For this review, take the finished solid that the model builds, in its own axes (mm). A direction names the side the tool comes from. Coordinates: 2 decimals unless noted, no trailing zeros. Loops run counter-clockwise (first coordinate to the right, second up) from the corner with the lowest first, then second, coordinate; pieces in that order, holes last.
1. To check wall thickness, follow probe 1 along Z at (x, y) = (-24.5, -33); probe 2 along Y at (x, z) = (27, 144.5); probe 3 along Y at (x, z) = (36, 93.5). State the ranges of each line that lie inside material, in increasing order.
2. Machinability: for faces 4 (the face through (-1, 1, 0)), 5 (the face through (32.364, 1.674, 147.451)), which of the approach directions +Z, -Z, +X, -X, +Y, -Y give a long, thin tool a straight path to every point of the face, cutting with its end or side? Answer none if there is none.
3. Take a section at B-B, the plane x = 26. State the section outline as (y, z) points, then the cut area to 3 significant figures.
4. Mouldability with a two-part tool opening along X and no side actions: class faces 1 (the face through (20.765, -39.923, 70.992)), 2 (the face through (-17.326, 1.696, 147.451)), 3 (the face through (-23, 0, 151)) as pulls with the +X half, pulls with the -X half, needs draft (parallel to the pull), parting line crosses it, or undercut.
5. Take a section at C-C, the plane z = 138. State the section outline as (x, y) points, then the cut area to 3 significant figures.
6. Take a section at D-D, the plane x = 0. State the section outline as (y, z) points, then the cut area to 3 significant figures.
7. Take a section at A-A, the plane y = 0. State the section outline as (x, z) points, then the cut area to 3 significant figures.
8. Clearance check with flat-ended pins moving along their axes: P1, Ø4, axis at x = 19.5, z = 22.5, coming from the +Y side; P2, Ø8, axis at x = -32.5, y = 33, coming from the -Z side; P3, Ø6, axis at x = 8, y = 11, coming from the +Z side; P4, Ø6, axis at x = 3, z = 18, coming from the -Y side. State where each tip first meets the part, or that it passes through.
```python
from build123d import *

# Parameters (mm, degrees)
SKETCH1_R           = 45
BOSS_EXTRUDE1_DEPTH = 144
SKETCH2_R           = 5.645084992
SKETCH2_R_2         = 5.573002613
BOSS_EXTRUDE2_DEPTH = 7


with BuildPart() as part:
    # Sketch1 → Boss-Extrude1 (new body)
    with BuildSketch(Plane.XY):
        Circle(SKETCH1_R)
    extrude(amount=BOSS_EXTRUDE1_DEPTH)

    # Sketch2 → Boss-Extrude2 (add)
    with BuildSketch(Plane.XY.offset(144)):
        with Locations((-22.710039741, 0)):
            Circle(SKETCH2_R)
        with Locations((27.048206136, 0)):
            Circle(SKETCH2_R_2)
    extrude(amount=BOSS_EXTRUDE2_DEPTH)


solid = part.part
```
Results list:
1. probe 1: z = 0 to 144
1. probe 2: y = -5.57 to 5.57
1. probe 3: y = -27 to 27
2. face 4: -Z, +X, -X, +Y, -Y
2. face 5: +Z
3. outline: (-36.73, 0) - (36.73, 0) - (36.73, 144) - (5.47, 144) - (5.47, 151) - (-5.47, 151) - (-5.47, 144) - (-36.73, 144) - close
3. area: 10,700 mm2
4. face 1: parting line crosses it
4. face 2: undercut
4. face 3: needs draft
5. outline: circle Ø90 at (0, 0)
5. area: 6,360 mm2
6. outline: (-45, 0) - (45, 0) - (45, 144) - (-45, 144) - close
6. area: 13,000 mm2
7. outline: (-45, 0) - (45, 0) - (45, 144) - (32.62, 144) - (32.62, 151) - (21.48, 151) - (21.48, 144) - (-17.06, 144) - (-17.06, 151) - (-28.36, 151) - (-28.36, 144) - (-45, 144) - close
7. area: 13,100 mm2
8. P1: stops at y = 41.46
8. P2: stops at z = 0
8. P3: stops at z = 144
8. P4: stops at y = -45
